The model under review builds one solid part; all positions refer to its coordinate system, in mm. Face numbers are marked on the shaded views. Coordinates: 2 decimals unless noted, no trailing zeros. Order: outer loops, then holes, each group sorted by start corner. A loop starts at its lowest first (then second) coordinate and runs counter-clockwise, first axis right, second up. Notation, with made-up numbers: M -13,2 L -6,2 A31 ccw -6,31 Z; hole C 47.5,-14.5 d5. An arc over 180 degrees is marked long. One line per item, written item: value.
```python
from build123d import *

# Parameters (mm, degrees)
SKETCH_1_R      = 0.5625
EXTRUDE_1_DEPTH = 1
FILLET_1_R      = 0.3
FILLET_2_R      = 0.3


with BuildPart() as part:
    # 草图1 → 凸台-拉伸1 (new body)
    with BuildSketch(Plane.XY):
        with BuildLine():
            Line((-0.75, 8.843253078), (-0.75, 5.448623679))
            ThreePointArc((-0.75, 5.448623679), (0, -5.5), (0.75, 5.448623679))
            Line((0.75, 5.448623679), (0.75, 8.843253078))
            ThreePointArc((0.75, 8.843253078), (1.890982428, 8.671205825), (3, 8.352581936))
            Line((3, 8.352581936), (3.185419652, 6.233225621))
            ThreePointArc((3.185419652, 6.233225621), (0, -7), (-3.185419652, 6.233225621))
            Line((-3.185419652, 6.233225621), (-3, 8.352581936))
            ThreePointArc((-3, 8.352581936), (-1.890982428, 8.671205825), (-0.75, 8.843253078))
        make_face()
        with Locations((-1.875, 7.145938379)):
            Circle(SKETCH_1_R, mode=Mode.SUBTRACT)
        with Locations(Location((1.875, 7.145938379, 0), (0, 0, 180))):
            Circle(SKETCH_1_R, mode=Mode.SUBTRACT)
    extrude(amount=EXTRUDE_1_DEPTH)

    # 圆角1
    fillet_1_edges = [part.edges().sort_by_distance(p)[0] for p in [
        (3, 8.352581936, 0.5),
        (-3, 8.352581936, 0.5),
    ]]
    fillet(fillet_1_edges, radius=FILLET_1_R)

    # 圆角2
    fillet_2_edges = [part.edges().sort_by_distance(p)[0] for p in [
        (3.185419652, 6.233225621, 0.5),
        (-3.185419652, 6.233225621, 0.5),
        (-0.75, 8.843253078, 0.5),
        (0.75, 8.843253078, 0.5),
    ]]
    fillet(fillet_2_edges, radius=FILLET_2_R)


solid = part.part
```
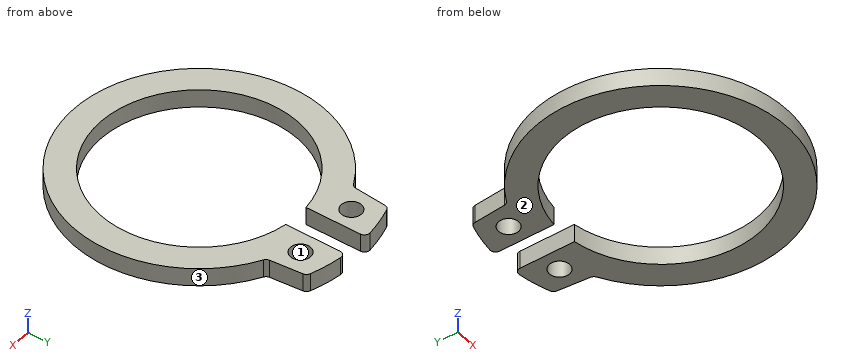
(1) We need section D-D, the plane x = 2. State the section outline as (y, z) points, plus the area to 3 significant figures.
Geometry results:
outline: M -6.71,0 L -5.12,0 L -5.12,1 L -6.71,1 Z; M 5.12,0 L 6.6,0 L 6.6,1 L 5.12,1 Z; M 7.69,0 L 8.65,0 L 8.65,1 L 7.69,1 Z
area: 4.01 mm2
(2) We need section B-B, the plane x = -4. State the section outline as (y, z) points.
Geometry results:
outline: M -5.74,0 L -3.77,0 L -3.77,1 L -5.74,1 Z; M 3.77,0 L 5.74,0 L 5.74,1 L 3.77,1 Z
(3) Mouldability with a two-part tool opening along X and no side actions: class the marked faces 1, 2 and 3 as +X half, -X half, draft (parallel to the pull), parting line (faces both ways), or undercut.
Geometry results:
face 1: undercut
face 2: draft
face 3: parting line
(4) We need section A-A, the plane y = 0. State the section outline as (x, z) points.
Geometry results:
outline: M -7,0 L -5.5,0 L -5.5,1 L -7,1 Z; M 5.5,0 L 7,0 L 7,1 L 5.5,1 Z
(5) Insertion check: pin 1 Ø0.5 at (y, z) = (6.5, 0.5) entering from +X. The pin has a flat end and moves straight along its axis. Give the tip position at first contact, or say it passes through.
Geometry results:
pin 1: stops at x = 3.22
(6) We need section C-C, the plane z = 0.6. Count the separate pieces of the cut face and the enclosed holes in it, plus the area to 3 significant figures.
Geometry results:
separate pieces: 1
enclosed holes: 2
area: 63.7 mm2
(7) For L1, parallel to X at y = 0, z = 0.45; L2, parallel to Y at x = 0, z = 0.6; L3, parallel to Y at x = 1.25, z = 0.15, list the stretches that pass through material, from the lowest coordinate up.
Geometry results:
L1: x = -7 to -5.5, 5.5 to 7
L2: y = -7 to -5.5
L3: y = -6.89 to -5.36, 5.36 to 8.79
